from build123d import *

# Parameters (mm, degrees)
F0_W     = 65
F0_H     = 9
F0_R     = 2.5
F1_DEPTH = 9
F2_DEPTH = 12.5
F3_W     = 7.776277
F3_H     = 9
F4_DEPTH = 25


with BuildPart() as f1:
    # F0 (on Front) → F1 (new body)
    with BuildSketch(Plane.XZ):
        with Locations((-32.5, 4.5)):
            Rectangle(F0_W, F0_H)
        with Locations((-57.5, 4.5)):
            Circle(F0_R, mode=Mode.SUBTRACT)
        with Locations((-7.5, 4.5)):
            Circle(F0_R, mode=Mode.SUBTRACT)
    extrude(amount=F1_DEPTH)

    # F0 (on Front) → F2 (join)
    with BuildSketch(Plane.XZ):
        with Locations((-57.5, 4.5)):
            Circle(F0_R)
        with Locations((-7.5, 4.5)):
            Circle(F0_R)
    extrude(amount=F2_DEPTH)

    # F3 (on face) → F4 (cut)
    with BuildSketch(Plane.YZ):
        with Locations((-12.888139, 4.5)):
            Rectangle(F3_W, F3_H)
    extrude(amount=-F4_DEPTH, mode=Mode.SUBTRACT)


solid = f1.part
Source: CAD feature listing. Evaluate the final solid. Frame: model axes, mm. A direction names the side the tool comes from. Round coordinates to 2 decimals unless told otherwise and drop trailing zeros. Loops run counter-clockwise (first coordinate to the right, second up) from the corner with the lowest first, then second, coordinate; pieces in that order, holes last. Notation, with made-up numbers: M 79,27 L 108,27 A18 ccw 108,48 Z; hole C 60,86 d2. An arc over 180 degrees is marked long. Answer as CSV lines item,"result".
Q1. Pull-direction query (Y, two-part tool) for faces 1 (the face through (-33, 0, 5)), 2 (the face through (-58, -12.5, 5)), 3 (the face through (0, -4, 4)); classes: +Y half, -Y half, draft (parallel to the pull), parting line (faces both ways), or undercut.
Verdict:
face 1,"+Y half"
face 2,"-Y half"
face 3,"draft"
Q2. Cut plane C-C (x = -40). Return the cut outline in (y, z).
Verdict:
outline,"M -9,0 L 0,0 L 0,9 L -9,9 Z"
Q3. Cut plane D-D (z = 8). Return the cut outline in (x, y).
Verdict:
outline,"M -65,-9 L 0,-9 L 0,0 L -65,0 Z"
Q4. Cut plane B-B (x = -57.5). Return the cut outline in (y, z).
Verdict:
outline,"M -12.5,2 L -9,2 L -9,0 L 0,0 L 0,9 L -9,9 L -9,7 L -12.5,7 Z"
Q5. Contact query for a flat-ended pin moving along its axis: pin 1 (5 mm diameter, centred on x = -37, z = 3.5, fed in from -Y). Output: stop coordinate, or through.
Verdict:
pin 1,"stops at y = -9"
Q6. Line query: line 1 along Y through (x, z) = (-55.5, 8). Output: solid intervals per line, ascending.
Verdict:
line 1,"y = -9 to 0"
Q7. Cut plane A-A (z = 4.5). Return the cut outline in (x, y), plus the area to 4 significant figures.
Verdict:
outline,"M -65,-9 L -60,-9 L -60,-12.5 L -55,-12.5 L -55,-9 L 0,-9 L 0,0 L -65,0 Z"
area,"602.5 mm^2"
Q8. Reachability of faces 4 (the face through (-33, -4, 9)), 5 (the face through (-55.19, -10.73, 3.54)) from +Z, -Z, +X, -X, +Y, -Y: full face, straight path, thin tool, end or side. Return the list, or none.
Verdict:
face 4,"+Z, +X, -X, +Y, -Y"
face 5,"-Y"
